Source: CAD feature listing. Evaluate the final solid. Frame: model axes, mm. Face numbers are marked on the shaded views. A direction names the side the tool comes from. Round coordinates to 2 decimals unless told otherwise and drop trailing zeros. Write each loop counter-clockwise with the first axis right and the second up, starting at its lowest first coordinate (ties: lowest second). Pieces come first, ordered by that corner, then holes. Notation, with made-up numbers: M 23.5,-30 L 39.5,-30 A8 cw 39.5,-23 Z; hole C 10,-6.5 d11. An arc over 180 degrees is marked long. Answer in a Markdown table with one row per item.
from build123d import *

# Parameters (mm, degrees)
BOSS_EXTRUDE1_DEPTH = 75
BOSS_EXTRUDE2_DEPTH = 24
CUT_EXTRUDE1_START  = 75
CUT_EXTRUDE1_DEPTH  = 36


with BuildPart() as part:
    # Sketch1 → Boss-Extrude1 (new body)
    with BuildSketch(Plane.XY):
        Polygon((25, 12), (9, 32), (0, 32), (0, 0), (50, 0), (50, 32), (41, 32), align=None)
        Polygon((32, 32), (9, 32), (25, 12), (41, 32), align=None)
    extrude(amount=BOSS_EXTRUDE1_DEPTH)

    # Sketch1<3> → Boss-Extrude2 (add)
    with BuildSketch(Plane.XY):
        Polygon((0, 32), (9, 32), (32, 32), (32, 56), (8, 56), align=None)
    extrude(amount=BOSS_EXTRUDE2_DEPTH)

    # Sketch1<4> → Cut-Extrude1 (cut)
    with BuildSketch(Plane.XY.offset(CUT_EXTRUDE1_START)):
        Polygon((32, 32), (9, 32), (25, 12), (41, 32), align=None)
    extrude(amount=-CUT_EXTRUDE1_DEPTH, mode=Mode.SUBTRACT)


solid = part.part
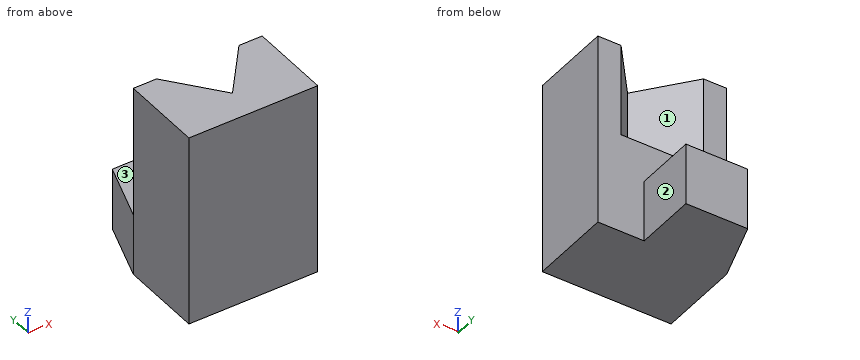
Q1. Material intervals for probe 1 along Y at (x, z) = (36.5, 29); probe 2 along Z at (x, y) = (15, 35); probe 3 along Z at (x, y) = (19, 24), sorted ascending.
Solutions:
| item | result |
|---|---|
| probe 1 | y = 0 to 32 |
| probe 2 | z = 0 to 24 |
| probe 3 | z = 0 to 39 |
Q2. Section C-C (y = 16). Return loops of the section in (x, z).
Solutions:
| item | result |
|---|---|
| outline | M 0,0 L 50,0 L 50,75 L 28.2,75 L 28.2,39 L 21.8,39 L 21.8,75 L 0,75 Z |
Q3. Contact query for flat-ended pins moving along their axis: pin 1 Ø7 at (x, y) = (10, 49) entering from +Z; pin 2 Ø6 at (x, z) = (19.5, 43) entering from +Y (3 decimals). Output: stop coordinate, or through.
Solutions:
| item | result |
|---|---|
| pin 1 | stops at z = 24 |
| pin 2 | stops at y = 22.625 |
Q4. Section B-B (z = 62). Return loops of the section in (x, y).
Solutions:
| item | result |
|---|---|
| outline | M 0,0 L 50,0 L 50,32 L 41,32 L 25,12 L 9,32 L 0,32 Z |
Q5. Section A-A (x = 31). Return loops of the section in (y, z), and give its area (3 significant figures).
Solutions:
| item | result |
|---|---|
| outline | M 0,0 L 56,0 L 56,24 L 32,24 L 32,39 L 19.5,39 L 19.5,75 L 0,75 Z |
| area | 2,530 mm2 |
Q6. Section D-D (z = 12). Return loops of the section in (x, y).
Solutions:
| item | result |
|---|---|
| outline | M 0,0 L 50,0 L 50,32 L 32,32 L 32,56 L 8,56 L 0,32 Z |
Q7. Access query for the marked faces 1, 2 and 3. Directions: +Z, -Z, +X, -X, +Y, -Y. A direction counts if a zero-diameter tool reaches every point of the face in a straight line with its end or side. Return the directions, or none.
Solutions:
| item | result |
|---|---|
| face 1 | +Z, +Y |
| face 2 | +Z, -Z, +X, +Y |
| face 3 | +Z, +X, -X, +Y |
